Geometry check sheet. Reference: the model listing, model coordinates, mm. A direction names the side the tool comes from. Coordinates: 2 decimals unless noted, no trailing zeros. Write each loop counter-clockwise with the first axis right and the second up, starting at its lowest first coordinate (ties: lowest second). Pieces come first, ordered by that corner, then holes. Notation, with made-up numbers: (41.5, 32) -> (52.5, 32) arc R24 cw to (52.5, 70) -> close; hole circle Ø8 at (-31.75, 64). An arc over 180 degrees is marked (long way). Answer as CSV lines item,"result".
```python
from build123d import *

# Parameters (mm, degrees)
SKETCH1_W           = 66
SKETCH1_H           = 50
BOSS_EXTRUDE1_DEPTH = 4
SKETCH2_W           = 4
SKETCH2_H           = 5
BOSS_EXTRUDE2_DEPTH = 4
LPATTERN1_COUNT     = 5
LPATTERN1_PITCH     = 10
SKETCH3_W           = 10
SKETCH3_H           = 4
BOSS_EXTRUDE3_DEPTH = 4
LPATTERN2_COUNT     = 2
LPATTERN2_PITCH     = 20
LPATTERN2_COL_COUNT = 2
LPATTERN2_COL_PITCH = 20
SKETCH4_W           = 10
SKETCH4_H           = 4
CUT_EXTRUDE1_DEPTH  = 87.116200566


with BuildPart() as part:
    # Sketch1 → Boss-Extrude1 (new body)
    with BuildSketch(Plane(origin=(0, 0, 0), x_dir=(1, 0, 0), z_dir=(0, 1, 0))):
        with Locations((33, -25)):
            Rectangle(SKETCH1_W, SKETCH1_H)
    extrude(amount=BOSS_EXTRUDE1_DEPTH)

    # Sketch2 → Boss-Extrude2 (add, through all)
    with BuildSketch(Plane(origin=(0, 4, 0), x_dir=(1, 0, 0), z_dir=(0, 1, 0))):
        with Locations((-2, -2.5)):
            Rectangle(SKETCH2_W, SKETCH2_H)
        with Locations((68, -2.5)):
            Rectangle(SKETCH2_W, SKETCH2_H)
    boss_extrude2 = extrude(amount=-BOSS_EXTRUDE2_DEPTH)

    # LPattern1: Boss-Extrude2 ×5
    with Locations(*[(0, 0, i * LPATTERN1_PITCH) for i in range(1, LPATTERN1_COUNT)]):
        add(boss_extrude2)

    # Sketch3 → Boss-Extrude3 (add, through all)
    with BuildSketch(Plane(origin=(0, 4, 0), x_dir=(1, 0, 0), z_dir=(0, 1, 0))):
        with Locations((33, 2)):
            Rectangle(SKETCH3_W, SKETCH3_H)
    boss_extrude3 = extrude(amount=-BOSS_EXTRUDE3_DEPTH)

    # LPattern2: Boss-Extrude3 ×2
    with Locations(*[(i * LPATTERN2_PITCH, 0, 0) for i in range(1, LPATTERN2_COUNT)]):
        add(boss_extrude3)

    # LPattern2 col: Boss-Extrude3 ×2
    with Locations(*[(-i * LPATTERN2_COL_PITCH, 0, 0) for i in range(1, LPATTERN2_COL_COUNT)]):
        add(boss_extrude3)

    # Sketch4 → Cut-Extrude1 (cut, through all)
    with BuildSketch(Plane.XZ):
        with Locations((13, 26)):
            Rectangle(SKETCH4_W, SKETCH4_H)
        with Locations((33, 26)):
            Rectangle(SKETCH4_W, SKETCH4_H)
        with Locations((53, 26)):
            Rectangle(SKETCH4_W, SKETCH4_H)
    extrude(amount=-CUT_EXTRUDE1_DEPTH, mode=Mode.SUBTRACT)


solid = part.part
```
Item 1: Cross-section at C-C, the plane y = 2.9. Count the separate pieces of the cut face and the enclosed holes in it, plus the area to 3 significant figures.
Responses:
separate pieces,"1"
enclosed holes,"3"
area,"3,500 mm2"
Item 2: Thickness scan on probe 1 along X at (y, z) = (2.1, 26); probe 2 along Z at (x, y) = (54.5, 1.75); probe 3 along X at (y, z) = (3.25, 37.5). Record the ranges inside material, lowest first.
Responses:
probe 1,"x = 0 to 8, 18 to 28, 38 to 48, 58 to 66"
probe 2,"z = -4 to 24, 28 to 50"
probe 3,"x = 0 to 66"
Item 3: Cross-section at B-B, the plane z = -1. Record the cut outline in (x, y).
Responses:
outline,"(8, 0) -> (18, 0) -> (18, 4) -> (8, 4) -> close; (28, 0) -> (38, 0) -> (38, 4) -> (28, 4) -> close; (48, 0) -> (58, 0) -> (58, 4) -> (48, 4) -> close"
Item 4: Release check for a two-part mould opening along X. For faces 4 (the flat face through (13, 2, 24)), 5 (the flat face through (33, 2, 50)), 6 (the flat face through (0, 2, 38)) record: +X half, -X half, draft (parallel to the pull), parting line (faces both ways), or undercut.
Responses:
face 4,"undercut"
face 5,"draft"
face 6,"-X half"
Item 5: Depth check by flat-ended pin: pin 1 Ø1.2 at (y, z) = (1, 25.5) entering from -X; pin 2 Ø2 at (y, z) = (1.5, -2) entering from -X; pin 3 Ø1.2 at (x, y) = (69, 3) entering from +Z; pin 4 Ø2 at (x, y) = (-2.5, 2.5) entering from -Z. Enter the tip coordinate at first touch or a pass-through.
Responses:
pin 1,"stops at x = -4"
pin 2,"stops at x = 8"
pin 3,"stops at z = 45"
pin 4,"stops at z = 0"
Item 6: Set-up check for faces 1 (the flat face through (66, 2, 48)), 2 (the flat face through (8, 2, -2)), 3 (the flat face through (0, 2, 28)): record each of +Z, -Z, +X, -X, +Y, -Y from which the full face is reachable in a straight line by a thin tool's end or side.
Responses:
face 1,"+Z, +X, +Y, -Y"
face 2,"-Z, -X, +Y, -Y"
face 3,"-X, +Y, -Y"
Item 7: Cross-section at A-A, the plane x = 29. Record the cut outline in (y, z).
Responses:
outline,"(0, -4) -> (4, -4) -> (4, 24) -> (0, 24) -> close; (0, 28) -> (4, 28) -> (4, 50) -> (0, 50) -> close"
Item 8: Cross-section at D-D, the plane x = 44. Record the cut outline in (y, z).
Responses:
outline,"(0, 0) -> (4, 0) -> (4, 50) -> (0, 50) -> close"
